Autodesk Inventor part; units mm, degrees
ref_plane "YZ Plane" through (0, 0, 0) normal (1, 0, 0) x (0, 1, 0)
ref_plane "XZ Plane" through (0, 0, 0) normal (0, 1, 0) x (-1, 0, 0)
ref_plane "XY Plane" through (0, 0, 0) normal (0, 0, 1) x (1, 0, 0)
sketch "Esquisse1" plane through (0, 0, 0) normal (0, 1, 0) x (-1, 0, 0)
  line L0 (-14.5, 51.941) -> (-10.5, 51.941)
  line L1 (-10.5, 51.941) -> (-10.5, -12.859)
  line L2 (-10.5, -12.859) -> (-14.5, -12.859)
  line L3 (-14.5, -12.859) -> (-14.5, 51.941)
  line L4 (10.5, 51.941) -> (14.5, 51.941)
  line L5 (14.5, 51.941) -> (14.5, -12.859)
  line L6 (14.5, -12.859) -> (10.5, -12.859)
  line L7 (10.5, -12.859) -> (10.5, 51.941)
  line L8 (-10.5, -6.459) -> (10.5, -6.459)
  line L9 (10.5, -6.459) -> (10.5, -12.859)
  line L10 (10.5, -12.859) -> (-10.5, -12.859)
  line L11 (-10.5, -12.859) -> (-10.5, -6.459)
  line L12 (-10.5, 41.941) -> (10.5, 41.941)
  line L13 (10.5, 41.941) -> (10.5, 35.541)
  line L14 (10.5, 35.541) -> (-10.5, 35.541)
  line L15 (-10.5, 35.541) -> (-10.5, 41.941)
  line L16 (10.5, -12.859) -> (14.5, -12.859)
  point P0 (0, 0)
  dimension "d1" = 6.4
  dimension "d2" = 21
  dimension "d3" = 4
  dimension "d4" = 4
  dimension "d5" = 10.5
  dimension "d6" = 42
  dimension "d7" = 10
  dimension "d8" = 35.541
  dimension "d9" = 6.4
extrude "Extrusion1" add sketch "Esquisse1" along normal blind 20 contours L0 L1 L2 L3 | L12 L7 L14 L1 | L1 L8 L7 L10 | L7 L4 L5 L6
sketch "Esquisse2" plane through (14.5, 0, 51.941) normal (1, 0, 0) x (0, 0, -1)
  line L0 (64.8, 0) -> (64.8, 20)
  line L1 (0, 0) -> (0, 20)
  line L2 (0, 10) -> (64.8, 10) construction
  circle A0 centre (14.8, 10) radius 3.5
  point P0 (51.941, 0)
  dimension "d12" = 50
  dimension "d13" = 7
extrude "Extrusion2" cut sketch "Esquisse2" against normal blind 3
sketch "Esquisse3" plane through (-14.5, 0, -12.859) normal (-1, 0, 0) x (0, 0, 1)
  line L0 (64.8, 0) -> (64.8, 20)
  line L1 (0, 0) -> (0, 20)
  line L2 (64.8, 10) -> (0, 10) construction
  circle A0 centre (50, 10) radius 3.5
  point P0 (12.859, 0)
  dimension "d16" = 50
  dimension "d17" = 7
extrude "Extrusion3" cut sketch "Esquisse3" against normal blind 3
sketch "Esquisse5" plane through (0, 20, 0) normal (0, 1, 0) x (1, 0, 0)
  line L0 (10.5, -35.541) -> (-10.5, -35.541)
  line L1 (14.5, 12.859) -> (-14.5, 12.859)
  line L2 (-10.5, -41.941) -> (10.5, -41.941)
  line L3 (-9.9, 12.859) -> (9.9, 12.859)
  line L4 (9.9, 12.859) -> (9.9, 6.459)
  line L5 (9.9, 6.459) -> (-9.9, 6.459)
  line L6 (-9.9, 6.459) -> (-9.9, 12.859)
  line L7 (-9.9, -41.941) -> (9.9, -41.941)
  line L8 (9.9, -41.941) -> (9.9, -35.541)
  line L9 (9.9, -35.541) -> (-9.9, -35.541)
  line L10 (-9.9, -35.541) -> (-9.9, -41.941)
  line L11 (0, 12.859) -> (0, -41.941)
  circle A0 centre (5, 9.659) radius 2.5
  circle A1 centre (5, -38.741) radius 2.5
  circle A2 centre (-5, 9.659) radius 2.5
  circle A3 centre (-5, -38.741) radius 2.5
  point P0 (0, 0)
  dimension "d29" = 6.4
  dimension "d30" = 6.4
  dimension "d31" = 19.8
  dimension "d32" = 9.9
  dimension "d33" = 5
  dimension "d34" = 5
  dimension "d35" = 5
  dimension "d36" = 5
  dimension "d37" = 3.2
  dimension "d38" = 3.2
extrude "Extrusion5" cut sketch "Esquisse5" against normal through all contours A0 | A1 | A2 | A3
sketch "Esquisse6" plane through (0, 20, 0) normal (0, 1, 0) x (1, 0, 0)
  circle A0 centre (-5, 9.659) radius 2.5
  circle A1 centre (5, 9.659) radius 2.5
  line L0 (14.5, -51.941) -> (14.5, 12.859)
  line L1 (-14.5, 12.859) -> (14.5, 12.859)
  line L2 (14.5, 12.859) -> (14.5, -17.141)
  line L3 (14.5, -17.141) -> (-14.5, -17.141)
  line L4 (-14.5, -17.141) -> (-14.5, 12.859)
  point P0 (0, 0)
  dimension "d41" = 30
extrude "Extrusion6" cut sketch "Esquisse6" against normal blind 15
chamfer "Chanfrein1" distance 15 angle 45 2 edges at (12.5, 20, 17.141) (-12.5, 20, 17.141)
fillet "Congé1" radius 3 2 edges at (-14.5, 2.5, -12.859) (14.5, 2.5, -12.859)
fillet "Congé2" radius 10 4 edges at (-12.5, 0, 51.941) (12.5, 0, 51.941) (-12.5, 20, 51.941) (12.5, 20, 51.941)
equation "\"d4\" = d3"
equation "\"d9\" = d1"
equation "\"d30\" = d29"
equation "\"d34\" = d33"
equation "\"d38\" = d37"
properties part number "new_shoulder_modified"
Here's how the part is built. I have some questions about the finished solid (model axes, mm). A direction names the side the tool comes from. Round coordinates to 2 decimals unless told otherwise and drop trailing zeros. Loops run counter-clockwise (first coordinate to the right, second up) from the corner with the lowest first, then second, coordinate; pieces in that order, holes last.
1. For P1, Ø3, axis at x = -1.5, y = 2.5, coming from the +Z side; P2, Ø3.5, axis at y = 10, z = 37.5, coming from the +X side; P3, Ø12, axis at x = -9, z = -3, coming from the +Y side, each with a flat end and sliding along its axis, tell me the tip position at first contact or that it passes through.
Answer list:
P1: stops at z = 41.94
P2: stops at x = 11.5
P3: stops at y = 5
2. If we section it at B-B on z = 6.5: Write out the boundary of the cut face in (x, y), plus the area to 3 significant figures.
Answer list:
outline: (-14.5, 0) - (-10.5, 0) - (-10.5, 5) - (-14.5, 5) - close; (10.5, 0) - (14.5, 0) - (14.5, 5) - (10.5, 5) - close
area: 40.0 mm2
3. If we section it at C-C on x = -5: Write out the boundary of the cut face in (y, z).
Answer list:
outline: (0, -12.86) - (5, -12.86) - (5, -12.16) - (0, -12.16) - close; (0, -7.16) - (5, -7.16) - (5, -6.46) - (0, -6.46) - close; (0, 35.54) - (20, 35.54) - (20, 36.24) - (0, 36.24) - close; (0, 41.24) - (20, 41.24) - (20, 41.94) - (0, 41.94) - close
4. If we section it at D-D on y = 11.5: Write out the boundary of the cut face in (x, z).
Answer list:
outline: (-14.5, 23.64) - (-10.5, 23.64) - (-10.5, 35.54) - (10.5, 35.54) - (10.5, 23.64) - (14.5, 23.64) - (14.5, 33.98) - (11.5, 33.98) - (11.5, 40.3) - (14.5, 40.3) - (14.5, 51.83) - (10.5, 51.83) - (10.5, 41.94) - (-10.5, 41.94) - (-10.5, 51.83) - (-14.5, 51.83) - (-14.5, 40.3) - (-11.5, 40.3) - (-11.5, 33.98) - (-14.5, 33.98) - close; hole circle Ø5 at (-5, 38.74); hole circle Ø5 at (5, 38.74)
5. If I drill on line 1 along Z through (x, y) = (5, 2.05); line 2 along X through (y, z) = (2, 43); line 3 along Z through (x, y) = (9.5, 4), over which ranges is the centre line in solid material (lowest first)?
Answer list:
line 1: z = -12.86 to -12.16, -7.16 to -6.46, 35.54 to 36.24, 41.24 to 41.94
line 2: x = -14.5 to -10.5, 10.5 to 14.5
line 3: z = -12.86 to -6.46, 35.54 to 41.94
6. Which directions (+Z, -Z, +X, -X, +Y, -Y) give clear straight access to the entire face, cutting with the end or side of a thin tool? Please do faces 4 (the face through (0, 10, 41.941)), 5 (the face through (13.02, 7.87, 39.92)), 6 (the face through (-13.021, 8.659, 40.374)), 7 (the face through (0, 10, 35.541)).
Answer list:
face 4: +Z, +Y, -Y
face 5: +X
face 6: -X
face 7: +Y, -Y
7. We'd pull the mould along Y, two halves only. Please class faces 1 (the face through (-11.5, 10, 37)), 2 (the face through (0, 5, -7)), 3 (the face through (-2.615, 10.14, 37.99)): +Y half, -Y half, draft (parallel to the pull), parting line (faces both ways), or undercut.
Answer list:
face 1: undercut
face 2: +Y half
face 3: draft
8. If we section it at A-A on x = -8.25: Write out the boundary of the cut face in (y, z).
Answer list:
outline: (0, -12.86) - (5, -12.86) - (5, -6.46) - (0, -6.46) - close; (0, 35.54) - (20, 35.54) - (20, 41.94) - (0, 41.94) - close
